The listing builds one solid part. Answer for the finished solid, in the listing's coordinates (mm). Face numbers are marked on the shaded views. A direction names the side the tool comes from. Coordinates: 2 decimals unless noted, no trailing zeros. Order: outer loops, then holes, each group sorted by start corner. A loop starts at its lowest first (then second) coordinate and runs counter-clockwise, first axis right, second up.
from build123d import *

# Parameters (mm, degrees)
F0_W         = 25.4
F0_H         = 25.4
F1_DEPTH     = 25.4
F2_R         = 3.175
F9_DEPTH     = 1.778
F3_R         = 3.175
F10_DEPTH    = 1.778
F4_R         = 3.175
F11_DEPTH    = 1.778
F5_R         = 3.175
F12_DEPTH    = 1.778
F6_R         = 3.175
F13_DEPTH    = 1.778
F7_R         = 3.175
F14_DEPTH    = 1.778
F8_R         = 3.175
F15_DEPTH    = 1.778
F16_T1_DEPTH = 50.8


# Not quite as in the source:
# - a fillet or chamfer that OpenCascade refuses, or shapes differently, is made with other operations: its cross-section is extruded or revolved along the edge and cut away or added


with BuildPart() as f1:
    # F0 (on Front) → F1 (new body)
    with BuildSketch(Plane.XZ):
        with Locations((-25.9571580286, 18.6469587497)):
            Rectangle(F0_W, F0_H)
    extrude(amount=F1_DEPTH)

    # F2 (on face) → F9 (cut)
    with BuildSketch(Plane.XZ.offset(25.4)):
        with Locations((-31.6721580286, 12.9319587497)):
            Circle(F2_R)
    extrude(amount=-F9_DEPTH, mode=Mode.SUBTRACT)

    # F3 (on face) → F10 (cut)
    with BuildSketch(Plane.XZ.offset(25.4)):
        with Locations((-20.2421580286, 24.3619587497)):
            Circle(F3_R)
    extrude(amount=-F10_DEPTH, mode=Mode.SUBTRACT)

    # F4 (on face) → F11 (cut)
    with BuildSketch(Plane.XY.offset(31.3469587497)):
        with Locations((-26.6341753304, -12.7)):
            Circle(F4_R)
    extrude(amount=-F11_DEPTH, mode=Mode.SUBTRACT)

    # F5 (on face) → F12 (cut)
    with BuildSketch(Plane(origin=(-38.6571580286, 0, 0), x_dir=(0, -1, 0), z_dir=(-1, 0, 0))):
        with Locations((16.7485739568, 23.0596062836)):
            Circle(F5_R)
        with Locations((16.7485739568, 14.0053418102)):
            Circle(F5_R)
        with Locations((6.985, 23.0596062836)):
            Circle(F5_R)
        with Locations((6.985, 14.0053418102)):
            Circle(F5_R)
    extrude(amount=-F12_DEPTH, mode=Mode.SUBTRACT)

    # F6 (on face) → F13 (cut)
    with BuildSketch(Plane.YZ.offset(-13.2571580286)):
        with Locations((-12.7, 18.6469587497)):
            Circle(F6_R)
        with Locations((-19.558, 11.7889587497)):
            Circle(F6_R)
        with Locations((-5.842, 25.5049587497)):
            Circle(F6_R)
    extrude(amount=-F13_DEPTH, mode=Mode.SUBTRACT)

    # F7 (on face) → F14 (cut)
    with BuildSketch(Plane(origin=(0, 0, 5.9469587497), x_dir=(1, 0, 0), z_dir=(0, 0, -1))):
        with Locations((-32.3071580286, 12.7)):
            Circle(F7_R)
        with Locations((-19.6071580286, 12.7)):
            Circle(F7_R)
        with Locations((-32.3071580286, 20.5331463367)):
            Circle(F7_R)
        with Locations((-32.3071580286, 3.81)):
            Circle(F7_R)
        with Locations((-19.6071580286, 3.81)):
            Circle(F7_R)
        with Locations((-19.6071580286, 20.8129025996)):
            Circle(F7_R)
    extrude(amount=-F14_DEPTH, mode=Mode.SUBTRACT)

    # F8 (on face) → F15 (cut)
    with BuildSketch(Plane(origin=(0, 0, 0), x_dir=(-1, 0, 0), z_dir=(0, 1, 0))):
        with Locations((25.9571580286, 19.88068223)):
            Circle(F8_R)
        with Locations((18.3371580286, 26.2669587497)):
            Circle(F8_R)
        with Locations((18.3371580286, 11.0269587497)):
            Circle(F8_R)
        with Locations((33.5771580286, 11.0269587497)):
            Circle(F8_R)
        with Locations((33.5771580286, 26.2669587497)):
            Circle(F8_R)
    extrude(amount=-F15_DEPTH, mode=Mode.SUBTRACT)

    # F16: fillet of radius 5.08 on 4 edges, made by hand

    # F16_s2 → F16_t1 (cut)
    with BuildSketch(Plane.XY.offset(-6.7530412503)):
        with BuildLine():
            ThreePointArc((-33.5771580286, -25.4), (-37.1692604771, -23.9121024484), (-38.6571580286, -20.32))
            Line((-38.6571580286, -20.32), (-38.6571580286, -25.4))
            Line((-38.6571580286, -25.4), (-33.5771580286, -25.4))
        make_face()
        with BuildLine():
            ThreePointArc((-13.2571580286, -20.32), (-14.7450555802, -23.9121024484), (-18.3371580286, -25.4))
            Line((-18.3371580286, -25.4), (-13.2571580286, -25.4))
            Line((-13.2571580286, -25.4), (-13.2571580286, -20.32))
        make_face()
        with BuildLine():
            ThreePointArc((-13.2571580286, -5.08), (-14.7450555802, -1.4878975516), (-18.3371580286, 0))
            Line((-18.3371580286, 0), (-13.2571580286, 0))
            Line((-13.2571580286, 0), (-13.2571580286, -5.08))
        make_face()
        with BuildLine():
            ThreePointArc((-33.5771580286, 0), (-37.1692604771, -1.4878975516), (-38.6571580286, -5.08))
            Line((-38.6571580286, -5.08), (-38.6571580286, 0))
            Line((-38.6571580286, 0), (-33.5771580286, 0))
        make_face()
    extrude(amount=F16_T1_DEPTH, mode=Mode.SUBTRACT)


solid = f1.part
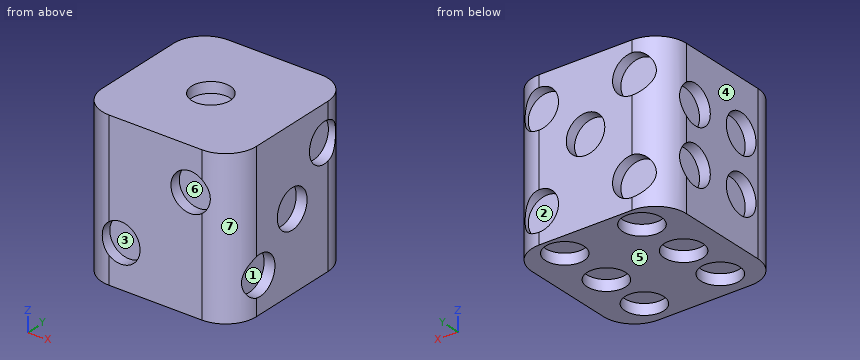
1) Consider L1, parallel to Y at x = -37, z = 23.5; L2, parallel to Z at x = -34, y = -2.75; L3, parallel to Z at x = -24.25, y = -14. Determine where each line is inside the solid, lowest interval first.
2) Section B-B (x = -25.25) is taken. Give the vertices of the cut face in (y, z), then the cut area to 3 significant figures.
3) A tool of negligible diameter and unlimited length cuts with its end or side. For the marked faces 1, 2 and 3, from which of +Z, -Z, +X, -X, +Y, -Y can it reach the whole face along a straight path? Write none if from no direction.
4) Section A-A (y = -12.7) is taken. Give the vertices of the cut face in (x, z).
5) Determine the mould class of the marked faces 4, 5, 6 and 7 for opening direction X: released by +X, released by -X, zero draft, split by the parting line, or undercut.
6) Each of these flat-tipped pins is pushed along its axis until it touches: P1, Ø3, axis at x = -20.5, y = -13, coming from the -Z side; P2, Ø5.5, axis at x = -26.63, y = -12.7, coming from the +Z side. Where does it stop, or does it pass through?
7) Section C-C (z = 23.5) is taken. Give the vertices of the cut face in (x, y), then the cut area to 3 significant figures.
8) Section D-D (y = -18.75) is taken. Give the vertices of the cut face in (x, z), then the cut area to 3 significant figures.
Filled sheet:
1. L1: y = -24.07 to -19.89, -13.6 to -10.13, -3.84 to -1.33
1. L2: z = 7.72 to 31.35
1. L3: z = 5.95 to 29.57
2. outline: (-25.4, 5.95) - (0, 5.95) - (0, 16.79) - (-1.78, 16.79) - (-1.78, 22.98) - (0, 22.98) - (0, 31.35) - (-9.84, 31.35) - (-9.84, 29.57) - (-15.56, 29.57) - (-15.56, 31.35) - (-25.4, 31.35) - close
2. area: 624 mm2
3. face 1: +X
3. face 2: +Y
3. face 3: -Y
4. outline: (-38.66, 5.95) - (-35.48, 5.95) - (-35.48, 7.72) - (-29.13, 7.72) - (-29.13, 5.95) - (-22.78, 5.95) - (-22.78, 7.72) - (-16.43, 7.72) - (-16.43, 5.95) - (-13.26, 5.95) - (-13.26, 15.47) - (-15.04, 15.47) - (-15.04, 21.82) - (-13.26, 21.82) - (-13.26, 31.35) - (-23.46, 31.35) - (-23.46, 29.57) - (-29.81, 29.57) - (-29.81, 31.35) - (-38.66, 31.35) - close
5. face 4: released by -X
5. face 5: zero draft
5. face 6: undercut
5. face 7: released by +X
6. P1: stops at z = 7.72
6. P2: stops at z = 29.57
7. outline: (-38.66, -20.32) arc R5.08 ccw to (-33.58, -25.4) - (-23.3, -25.4) - (-23.3, -23.62) - (-17.19, -23.62) - (-17.19, -25.27) arc R5.08 ccw to (-13.26, -20.32) - (-13.26, -8.3) - (-15.04, -8.3) - (-15.04, -3.38) - (-13.55, -3.38) arc R5.08 ccw to (-16.78, -0.24) - (-16.78, -1.78) - (-19.89, -1.78) - (-19.89, 0) - (-32.02, 0) - (-32.02, -1.78) - (-35.13, -1.78) - (-35.13, -0.24) arc R5.08 ccw to (-38.5, -3.84) - (-36.88, -3.84) - (-36.88, -10.13) - (-38.66, -10.13) - (-38.66, -13.6) - (-36.88, -13.6) - (-36.88, -19.89) - (-38.66, -19.89) - close
7. area: 570 mm2
8. outline: (-38.66, 5.95) - (-34.93, 5.95) - (-34.93, 7.72) - (-29.68, 7.72) - (-29.68, 5.95) - (-22.02, 5.95) - (-22.02, 7.72) - (-17.19, 7.72) - (-17.19, 5.95) - (-13.26, 5.95) - (-13.26, 8.72) - (-15.04, 8.72) - (-15.04, 14.86) - (-13.26, 14.86) - (-13.26, 31.35) - (-38.66, 31.35) - (-38.66, 25.52) - (-36.88, 25.52) - (-36.88, 20.59) - (-38.66, 20.59) - (-38.66, 16.47) - (-36.88, 16.47) - (-36.88, 11.54) - (-38.66, 11.54) - close
8. area: 599 mm2
